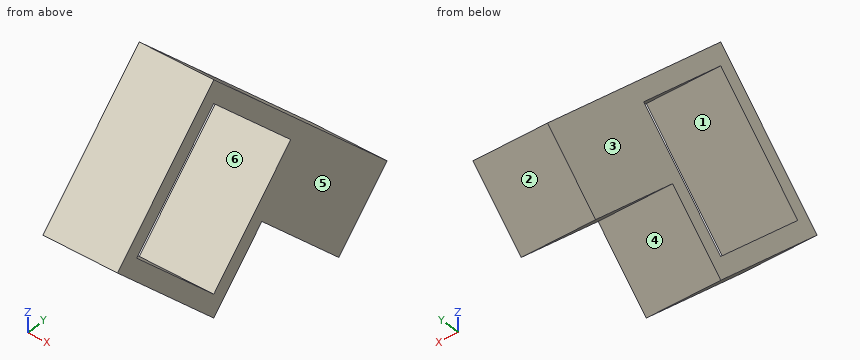
from build123d import *

# Parameters (mm, degrees)
EXTRUDE_1_DEPTH     = 20
CUT_EXTRUDE_1_DEPTH = 20


with BuildPart() as part:
    # 草图2 → 凸台-拉伸1 (new body)
    with BuildSketch(Plane(origin=(0, 0, 0), x_dir=(0, 0, -1), z_dir=(1, 0, 0))):
        Polygon((0, -31.819805153), (31.819805153, 0), (15.909902577, 15.909902577), (41.365746699, 41.365746699), (25.455844123, 57.275649276), (-15.909902577, 15.909902577), (-31.819805153, 0), align=None)
    extrude(amount=EXTRUDE_1_DEPTH)

    # 草图3 → 切除-拉伸1 (cut)
    with BuildSketch(Plane(origin=(20, 0, 0), x_dir=(0, 0, -1), z_dir=(1, 0, 0))):
        Polygon((0, -25.455844123), (25.455844123, 0), (0, 25.455844123), (-25.455844123, 0), align=None)
    extrude(amount=-CUT_EXTRUDE_1_DEPTH, mode=Mode.SUBTRACT)


solid = part.part
The listing builds one solid part. Answer for the finished solid, in the listing's coordinates (mm). Face numbers are marked on the shaded views. A direction names the side the tool comes from. Give positions to 0.01 mm unless a question says otherwise; leave off trailing zeros. Loops run counter-clockwise (first coordinate to the right, second up) from the corner with the lowest first, then second, coordinate; pieces in that order, holes last. Notation, with made-up numbers: M 32.25,63 L 88.25,63 A11 cw 88.25,84 Z; hole C -14.5,-6.75 d3. An arc over 180 degrees is marked long. Answer as CSV lines item,"result".
Item 1: Straight lines are drawn through the part: line 1 along Y through (x, z) = (15.25, -22.5); line 2 along Y through (x, z) = (17.25, 1.5); line 3 along Y through (x, z) = (9.5, -13). For each, find the intervals that lie inside material, in ascending order. Write a range as [from, to].
Values follow:
line 1,"y = [-9.32, -2.96], [2.96, 9.32], [22.5, 54.32]"
line 2,"y = [-30.32, -23.96], [23.96, 30.32]"
line 3,"y = [-18.82, -12.46], [12.46, 44.82]"
Item 2: The part is cut by section B-B (x = 5.5). Give the vertices of the cut face in (y, z), and give its area (3 significant figures).
Values follow:
outline,"M -31.82,0 L 0,-31.82 L 15.91,-15.91 L 41.37,-41.37 L 57.28,-25.46 L 0,31.82 Z; hole M -25.46,0 L 0,-25.46 L 25.46,0 L 0,25.46 Z"
area,"1,540 mm^2"
Item 3: The part is cut by section D-D (z = -21.5). Give the vertices of the cut face in (x, y), and give its area (3 significant figures).
Values follow:
outline,"M 0,-10.32 L 20,-10.32 L 20,-3.96 L 0,-3.96 Z; M 0,3.96 L 20,3.96 L 20,10.32 L 0,10.32 Z; M 0,21.5 L 20,21.5 L 20,53.32 L 0,53.32 Z"
area,"891 mm^2"
Item 4: Given pin 1 Ø12 at (x, y) = (7, 43.5) entering from +Z; pin 2 Ø3 at (x, z) = (17, -4.5) entering from -Y; pin 3 Ø10 at (x, y) = (5.5, 26) entering from -Z; pin 4 Ø5 at (y, z) = (-17, 16) entering from +X, each flat-ended and moving along its own axis, determine where each tip first touches the part or whether it passes through.
Values follow:
pin 1,"stops at z = -5.68"
pin 2,"stops at y = -28.82"
pin 3,"stops at z = -31"
pin 4,"stops at x = 20"
Item 5: The part is cut by section C-C (z = -11.5). Give the vertices of the cut face in (x, y), and give its area (3 significant figures).
Values follow:
outline,"M 0,-20.32 L 20,-20.32 L 20,-13.96 L 0,-13.96 Z; M 0,13.96 L 20,13.96 L 20,43.32 L 0,43.32 Z"
area,"715 mm^2"
Item 6: The part is cut by section A-A (y = 12). Give the vertices of the cut face in (x, z), and give its area (3 significant figures).
Values follow:
outline,"M 0,-19.82 L 20,-19.82 L 20,-13.46 L 0,-13.46 Z; M 0,13.46 L 20,13.46 L 20,19.82 L 0,19.82 Z"
area,"255 mm^2"
Item 7: Which of the six approach directions +Z, -Z, +X, -X, +Y, -Y give full straight-line access (tool end or side, diameter ignored) to the marked faces 4, 5 and 6?
Values follow:
face 4,"-Z, +X, -X"
face 5,"+Z, -Z, +X, +Y, -Y"
face 6,"+X, -X"
Item 8: The mould has two halves that part along Y. Classify the marked faces 1, 2 and 3: released by +Y, released by -Y, zero draft, split by the parting line, or undercut.
Values follow:
face 1,"undercut"
face 2,"released by +Y"
face 3,"zero draft"
